Could you check a few things on this drawing? It's one solid part, dimensions in mm from its lowest x, y, z. A direction names the side the tool comes from. Round coordinates to 2 decimals unless told otherwise and drop trailing zeros. Order: outer loops, then holes, each group sorted by start corner. A loop starts at its lowest first (then second) coordinate and runs counter-clockwise, first axis right, second up. Notation, with made-up numbers: (19.5, 69.5) -> (61.5, 69.5) arc R20 cw to (61.5, 84.5) -> close; hole circle Ø1 at (3, 38). An arc over 180 degrees is marked (long way). Use a Markdown table: item, result. Add a question column.
(1) I want a section at B-B, the plane x = 18.5. Please give me the cut outline in (y, z), then the cut area to 3 significant figures.
(2) I'm going to push flat-ended pins straight in: P1, Ø1, axis at x = 29, z = 56, coming from the -Y side; P2, Ø15, axis at x = 119.5, y = 25, coming from the +Z side; P3, Ø7.5, axis at y = 87.5, z = 88.5, coming from the +X side. Where does each tip first touch, or does it pass through?
(3) I want a section at D-D, the plane x = 43. Please give me the cut outline in (y, z), then the cut area to 3 significant figures.
(4) Thinking about a two-plate mould opening in X: for the marked faces 1, 2, 3 and 4, which applies, pulls with the +X half, pulls with the -X half, needs draft (parallel to the pull), parting line crosses it, or undercut?
(5) If I drill on probe 1 along Y at (x, z) = (119, 29); probe 2 along Z at (x, y) = (150, 85); probe 3 along Z at (x, y) = (86, 22), over which ranges is the centre line in solid material (lowest first)?
(6) On a 3-axis mill with a long thin cutter (end or side, diameter ignored), from which of +Z, -Z, +X, -X, +Y, -Y can I reach the whole of each face in a straight line? I mean the marked faces 5 and 6. Say none if no direction works.
(7) I want a section at C-C, the plane y = 69.5. Please give me the cut outline in (x, z), then the cut area to 3 significant figures.
(8) I want a section at A-A, the plane z = 94.5. Please give me the cut outline in (x, y).
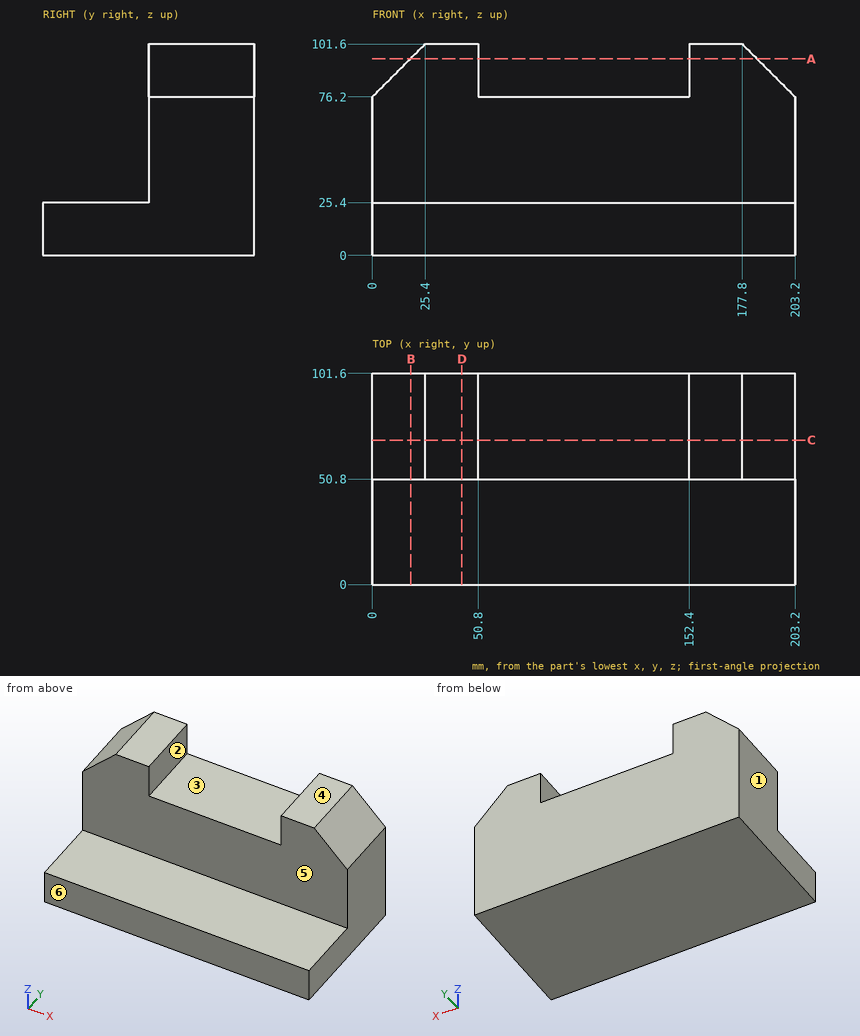
Taken from the geometry:
| question | item | result |
|---|---|---|
| 1 | outline | (0, 0) -> (101.6, 0) -> (101.6, 94.7) -> (50.8, 94.7) -> (50.8, 25.4) -> (0, 25.4) -> close |
| 1 | area | 6,100 mm2 |
| 2 | P1 | stops at y = 50.8 |
| 2 | P2 | stops at z = 25.4 |
| 2 | P3 | stops at x = 194.65 |
| 3 | outline | (0, 0) -> (101.6, 0) -> (101.6, 101.6) -> (50.8, 101.6) -> (50.8, 25.4) -> (0, 25.4) -> close |
| 3 | area | 6,450 mm2 |
| 4 | face 1 | pulls with the -X half |
| 4 | face 2 | undercut |
| 4 | face 3 | undercut |
| 4 | face 4 | needs draft |
| 5 | probe 1 | y = 50.8 to 101.6 |
| 5 | probe 2 | z = 0 to 76.2 |
| 5 | probe 3 | z = 0 to 25.4 |
| 6 | face 5 | +Z, +X, -X, -Y |
| 6 | face 6 | +Z, -Z, +X, -X, -Y |
| 7 | outline | (0, 0) -> (203.2, 0) -> (203.2, 76.2) -> (177.8, 101.6) -> (152.4, 101.6) -> (152.4, 76.2) -> (50.8, 76.2) -> (50.8, 101.6) -> (25.4, 101.6) -> (0, 76.2) -> close |
| 7 | area | 17,400 mm2 |
| 8 | outline | (18.3, 50.8) -> (50.8, 50.8) -> (50.8, 101.6) -> (18.3, 101.6) -> close; (152.4, 50.8) -> (184.9, 50.8) -> (184.9, 101.6) -> (152.4, 101.6) -> close |
